from build123d import *

# Parameters (mm, degrees)
F0_R     = 1.9304
F0_R_2   = 4
F1_DEPTH = 9.525
F2_SIZE  = 3.81
F3_R     = 4.5
F4_DEPTH = 3.81


with BuildPart() as f1:
    # F0 (on Right) → F1 (new body)
    with BuildSketch(Plane.YZ):
        with BuildLine():
            ThreePointArc((-25.373425, 125.624167), (-34.353681, 121.904423), (-38.073425, 112.924167))
            Line((-38.073425, 112.924167), (-38.073425, -99.800833))
            ThreePointArc((-38.073425, -99.800833), (-34.353681, -108.781089), (-25.373425, -112.500833))
            Line((-25.373425, -112.500833), (0.026575, -112.500833))
            Line((0.026575, -112.500833), (25.426575, -112.500833))
            ThreePointArc((25.426575, -112.500833), (34.406831, -108.781089), (38.126575, -99.800833))
            Line((38.126575, -99.800833), (38.126575, 112.924167))
            ThreePointArc((38.126575, 112.924167), (34.406831, 121.904423), (25.426575, 125.624167))
            Line((25.426575, 125.624167), (0.026575, 125.624167))
            Line((0.026575, 125.624167), (-25.373425, 125.624167))
        make_face()
        with Locations((0, -102.975833)):
            Circle(F0_R, mode=Mode.SUBTRACT)
        with Locations((-9.525, -54.732225)):
            Circle(F0_R_2, mode=Mode.SUBTRACT)
        with Locations((0, -70.430465)):
            Circle(F0_R_2, mode=Mode.SUBTRACT)
        with Locations((-23.624859, -45.638193)):
            Circle(F0_R_2, mode=Mode.SUBTRACT)
        with Locations((-9.525, -31.538333)):
            Circle(F0_R_2, mode=Mode.SUBTRACT)
        with Locations((-9.525, -12.488333)):
            Circle(F0_R_2, mode=Mode.SUBTRACT)
        with Locations((-9.525, 6.561667)):
            Circle(F0_R_2, mode=Mode.SUBTRACT)
        with Locations((9.525, -54.732225)):
            Circle(F0_R_2, mode=Mode.SUBTRACT)
        with Locations((9.525, -31.538333)):
            Circle(F0_R_2, mode=Mode.SUBTRACT)
        with Locations((9.525, -12.488333)):
            Circle(F0_R_2, mode=Mode.SUBTRACT)
        with Locations((9.525, 6.561667)):
            Circle(F0_R_2, mode=Mode.SUBTRACT)
        with Locations((23.624859, -45.638193)):
            Circle(F0_R_2, mode=Mode.SUBTRACT)
        with Locations((-23.624859, 58.761526)):
            Circle(F0_R_2, mode=Mode.SUBTRACT)
        with Locations((-9.525, 25.611667)):
            Circle(F0_R_2, mode=Mode.SUBTRACT)
        with Locations((-9.525, 44.661667)):
            Circle(F0_R_2, mode=Mode.SUBTRACT)
        with Locations((-9.525, 67.855558)):
            Circle(F0_R_2, mode=Mode.SUBTRACT)
        with Locations((0, 83.553798)):
            Circle(F0_R_2, mode=Mode.SUBTRACT)
        with Locations((0, 116.099167)):
            Circle(F0_R, mode=Mode.SUBTRACT)
        with Locations((9.525, 25.611667)):
            Circle(F0_R_2, mode=Mode.SUBTRACT)
        with Locations((9.525, 44.661667)):
            Circle(F0_R_2, mode=Mode.SUBTRACT)
        with Locations((23.624859, 58.761526)):
            Circle(F0_R_2, mode=Mode.SUBTRACT)
        with Locations((9.525, 67.855558)):
            Circle(F0_R_2, mode=Mode.SUBTRACT)
    extrude(amount=F1_DEPTH)

    # F2
    f2_edges = [f1.edges().sort_by_distance(p)[0] for p in [
        (9.525, -4, 83.553798),
        (9.525, 5.525, 67.855558),
        (9.525, 19.624859, 58.761526),
        (9.525, -13.525, 67.855558),
        (9.525, -27.624859, 58.761526),
        (9.525, -13.525, 44.661667),
        (9.525, 5.525, 44.661667),
        (9.525, -13.525, 25.611667),
        (9.525, -13.525, 6.561667),
        (9.525, -13.525, -12.488333),
        (9.525, -13.525, -31.538333),
        (9.525, 5.525, -31.538333),
        (9.525, 5.525, -12.488333),
        (9.525, 5.525, 6.561667),
        (9.525, 5.525, 25.611667),
        (9.525, 19.624859, -45.638193),
        (9.525, 5.525, -54.732225),
        (9.525, -13.525, -54.732225),
        (9.525, -27.624859, -45.638193),
        (9.525, -4, -70.430465),
    ]]
    chamfer(f2_edges, length=F2_SIZE)

    # F3 (on Right) → F4 (cut)
    with BuildSketch(Plane.YZ):
        with Locations((0, -70.430465)):
            Circle(F3_R)
        with Locations((0, 83.553798)):
            Circle(F3_R)
        with Locations((9.525, -31.538333)):
            Circle(F3_R)
        with Locations((9.525, -12.488333)):
            Circle(F3_R)
        with Locations((9.525, 6.561667)):
            Circle(F3_R)
        with Locations((9.525, 25.611667)):
            Circle(F3_R)
        with Locations((9.525, 44.661667)):
            Circle(F3_R)
        with Locations((-9.525, -31.538333)):
            Circle(F3_R)
        with Locations((-9.525, -12.488333)):
            Circle(F3_R)
        with Locations((-9.525, 6.561667)):
            Circle(F3_R)
        with Locations((-9.525, 25.611667)):
            Circle(F3_R)
        with Locations((-9.525, 44.661667)):
            Circle(F3_R)
        with Locations((23.624859, 58.761526)):
            Circle(F3_R)
        with Locations((9.525, 67.855558)):
            Circle(F3_R)
        with Locations((-23.624859, 58.761526)):
            Circle(F3_R)
        with Locations((-9.525, 67.855558)):
            Circle(F3_R)
        with Locations((23.624859, -45.638193)):
            Circle(F3_R)
        with Locations((9.525, -54.732225)):
            Circle(F3_R)
        with Locations((-9.525, -54.732225)):
            Circle(F3_R)
        with Locations((-23.624859, -45.638193)):
            Circle(F3_R)
    extrude(amount=F4_DEPTH, mode=Mode.SUBTRACT)


solid = f1.part
Input: part model. Units: mm. Frame: model coordinates. A direction names the side the tool comes from. Give positions to 0.01 mm unless a question says otherwise; leave off trailing zeros.
Q1. Draft query along Y for faces 1 (the flat face through (5, 0, -112.501)), 2 (the conical face through (5.95, 8.61, -58.87)), 3 (the cylindrical face through (4.749, -7.679, 64.307)). Return one class per face: +Y half, -Y half, draft (parallel to the pull), parting line (faces both ways), or undercut.
Checked values:
face 1: draft
face 2: undercut
face 3: undercut
Q2. Section A-A on x = 2.25. State how many separate pieces and enclosed holes the cut face has, and give its area (3 significant figures).
Checked values:
separate pieces: 1
enclosed holes: 22
area: 16,700 mm2
Q3. Contact query for flat-ended pins moving along their axis: pin 1 Ø9 at (y, z) = (23.62, -45.64) entering from +X; pin 2 Ø14.5 at (y, z) = (-9.52, 44.66) entering from +X; pin 3 Ø2.5 at (y, z) = (11.5, 45) entering from -X; pin 4 Ø10.5 at (y, z) = (9.52, 67.86) entering from +X. Output: stop coordinate, or through.
Checked values:
pin 1: stops at x = 6.22
pin 2: stops at x = 8.97
pin 3: passes through
pin 4: stops at x = 6.97
Q4. Ray query, probe 1 along Y at (x, z) = (1.75, 70); probe 2 along Z at (x, y) = (4.5, 0); probe 3 along Z at (x, y) = (2.4, 0). Return the intervals inside material, ascending.
Checked values:
probe 1: y = -38.07 to -13.48, -5.57 to 5.57, 13.48 to 38.13
probe 2: z = -112.5 to -104.91, -101.05 to -74.43, -66.43 to 79.55, 87.55 to 114.17, 118.03 to 125.62
probe 3: z = -112.5 to -104.91, -101.05 to -74.93, -65.93 to 79.05, 88.05 to 114.17, 118.03 to 125.62
Q5. Set-up query: faces 4 (the cylindrical face through (1.878, 11.944, -50.938)), 5 (the conical face through (5.95, -10.44, 63.72)). Return all of +Z, -Z, +X, -X, +Y, -Y with unobstructed straight access to the full face (end or side cutting, diameter ignored); none if empty.
Checked values:
face 4: -X
face 5: +X
